```python
from build123d import *

# Parameters (mm, degrees)
SKETCH1_W           = 25.5
SKETCH1_H           = 4
BOSS_EXTRUDE1_DEPTH = 2
FILLET1_R           = 10
SKETCH2_R           = 1.5
CUT_EXTRUDE1_DEPTH  = 53.603569832
SKETCH3_W           = 29.5
SKETCH3_H           = 2
BOSS_EXTRUDE2_DEPTH = 5.1
SKETCH4_W           = 29.5
SKETCH4_H           = 3
BOSS_EXTRUDE3_DEPTH = 13.8
SKETCH5_W           = 29.5
SKETCH5_H           = 2
BOSS_EXTRUDE5_DEPTH = 34.8
SKETCH7_W           = 29.5
SKETCH7_H           = 2
BOSS_EXTRUDE6_DEPTH = 13.8
SKETCH8_W           = 2
SKETCH8_H           = 4
SKETCH8_H_2         = 6.1
BOSS_EXTRUDE7_DEPTH = 12
SKETCH9_2_R         = 1.25
CUT_EXTRUDE3_DEPTH  = 12
SKETCH9_R           = 1.25
CUT_EXTRUDE2_DEPTH  = 12


with BuildPart() as part:
    # Sketch1 → Boss-Extrude1 (new body)
    with BuildSketch(Plane(origin=(0, 0, 0), x_dir=(1, 0, 0), z_dir=(0, 1, 0))):
        Polygon((-37.234375, 16.8984375), (-41.234375, 16.8984375), (-41.234375, -32.6015625), (-37.234375, -32.6015625), (-37.234375, 12.8984375), align=None)
        with Locations((-24.484375, 14.8984375)):
            Rectangle(SKETCH1_W, SKETCH1_H)
    extrude(amount=BOSS_EXTRUDE1_DEPTH)

    # Fillet1
    fillet1_edges = [part.edges().sort_by_distance(p)[0] for p in [
        (-37.234375, 1, -12.8984375),
    ]]
    fillet(fillet1_edges, radius=FILLET1_R)

    # Sketch2 → Cut-Extrude1 (cut, through all)
    with BuildSketch(Plane(origin=(0, 2, 0), x_dir=(1, 0, 0), z_dir=(0, 1, 0))):
        with Locations(Location((-38.984375, -30.3515625, 0), (0, 0, 270))):
            Circle(SKETCH2_R)
        with Locations(Location((-38.984375, 14.6484375, 0), (0, 0, 270))):
            Circle(SKETCH2_R)
        with Locations(Location((-13.984375, 14.6484375, 0), (0, 0, 270))):
            Circle(SKETCH2_R)
    extrude(amount=-CUT_EXTRUDE1_DEPTH, mode=Mode.SUBTRACT)

    # Sketch3 → Boss-Extrude2 (add)
    with BuildSketch(Plane(origin=(0, 0, -16.8984375), x_dir=(-1, 0, 0), z_dir=(0, 0, -1))):
        with Locations((26.484375, 1)):
            Rectangle(SKETCH3_W, SKETCH3_H)
    extrude(amount=BOSS_EXTRUDE2_DEPTH)

    # Sketch4 → Boss-Extrude3 (add)
    with BuildSketch(Plane.XZ):
        with Locations((-26.484375, -20.4984375)):
            Rectangle(SKETCH4_W, SKETCH4_H)
    extrude(amount=BOSS_EXTRUDE3_DEPTH)

    # Sketch5 → Boss-Extrude5 (add)
    with BuildSketch(Plane(origin=(0, 0, -21.9984375), x_dir=(-1, 0, 0), z_dir=(0, 0, -1))):
        with Locations((26.484375, -12.8)):
            Rectangle(SKETCH5_W, SKETCH5_H)
    extrude(amount=BOSS_EXTRUDE5_DEPTH)

    # Sketch7 → Boss-Extrude6 (add)
    with BuildSketch(Plane(origin=(0, -11.8, 0), x_dir=(1, 0, 0), z_dir=(0, 1, 0))):
        with Locations((-26.484375, 55.7984375)):
            Rectangle(SKETCH7_W, SKETCH7_H)
    extrude(amount=BOSS_EXTRUDE6_DEPTH)

    # Sketch8 → Boss-Extrude7 (add)
    with BuildSketch(Plane(origin=(0, -11.8, 0), x_dir=(1, 0, 0), z_dir=(0, 1, 0))):
        with Locations((-12.734375, 23.9984375)):
            Rectangle(SKETCH8_W, SKETCH8_H)
        with Locations((-12.734375, 51.7484375)):
            Rectangle(SKETCH8_W, SKETCH8_H_2)
    extrude(amount=BOSS_EXTRUDE7_DEPTH)

    # Sketch9_2 → Cut-Extrude3 (cut)
    with BuildSketch(Plane(origin=(-11.734375, 0, 0), x_dir=(0, 0, -1), z_dir=(1, 0, 0))):
        with Locations((23.4984375, -5.55)):
            Circle(SKETCH9_2_R)
        with Locations((51.1984375, -5.55)):
            Circle(SKETCH9_2_R)
    extrude(amount=-CUT_EXTRUDE3_DEPTH, mode=Mode.SUBTRACT)

    # Sketch9 → Cut-Extrude2 (cut)
    with BuildSketch(Plane(origin=(-11.734375, 0, 0), x_dir=(0, 0, -1), z_dir=(1, 0, 0))):
        with Locations((23.4984375, -5.55)):
            Circle(SKETCH9_R)
        with Locations((51.1984375, -5.55)):
            Circle(SKETCH9_R)
    extrude(amount=-CUT_EXTRUDE2_DEPTH, mode=Mode.SUBTRACT)


solid = part.part
```
The listing builds one solid part. Answer for the finished solid, in the listing's coordinates (mm). A direction names the side the tool comes from. Round coordinates to 2 decimals unless told otherwise and drop trailing zeros. Loops run counter-clockwise (first coordinate to the right, second up) from the corner with the lowest first, then second, coordinate; pieces in that order, holes last. Notation, with made-up numbers: (-19, -3) -> (29, -3) arc R14 cw to (29, 15) -> close; hole circle Ø4 at (86.5, -17). An arc over 180 degrees is marked (long way). Use one line per item in the form item = value.
1. The part is cut by section D-D on x = -28.75. Determine the outline of the cut face in (y, z), and give its area (3 significant figures).
Answer key:
outline = (-13.8, -56.8) -> (2, -56.8) -> (2, -54.8) -> (-11.8, -54.8) -> (-11.8, -22) -> (2, -22) -> (2, -12.78) -> (0, -12.78) -> (0, -19) -> (-13.8, -19) -> close
area = 157 mm²
2. The part is cut by section C-C on z = -32. Determine the outline of the cut face in (x, y).
Answer key:
outline = (-41.23, -13.8) -> (-11.73, -13.8) -> (-11.73, -11.8) -> (-41.23, -11.8) -> close
3. Flat-ended cylindrical pins translate along their axes: pin 1 Ø3.5 at (x, z) = (-13.98, -14.65) entering from -Y; pin 2 Ø1.6 at (x, y) = (-19.5, 1.5) entering from +Z; pin 3 Ø0.6 at (x, y) = (-12.5, -4.5) entering from +Z. Find the tip coordinate at first contact, or state that the pin passes through.
Answer key:
pin_1 = 0
pin_2 = -12.9
pin_3 = -19
4. The part is cut by section A-A on y = -8.75. Determine the outline of the cut face in (x, z), and give its area (3 significant figures).
Answer key:
outline = (-41.23, -56.8) -> (-11.73, -56.8) -> (-11.73, -48.7) -> (-13.73, -48.7) -> (-13.73, -54.8) -> (-41.23, -54.8) -> close; (-41.23, -22) -> (-13.73, -22) -> (-13.73, -26) -> (-11.73, -26) -> (-11.73, -19) -> (-41.23, -19) -> close
area = 168 mm²
5. Find the intervals of material crossed by probe 1 along Z at (x, y) = (-33, -4); probe 2 along Y at (x, z) = (-34, -15), in increasing order. Write a range as [from, to].
Answer key:
probe_1 = [-56.8, -54.8], [-22, -19]
probe_2 = [0, 2]
6. For a pull along Z with two mould halves and no side action, classify faces 1 (the flat face through (-13.734, -6, -25)), 2 (the flat face through (-41.234, -4.2, -21.8)), 3 (the flat face through (-27, -6, -56.798)), 4 (the cylindrical face through (-34.383, 1.014, -9.891)) as released by +Z, released by -Z, zero draft, split by the parting line, or undercut.
Answer key:
face_1 = undercut
face_2 = zero draft
face_3 = released by -Z
face_4 = released by +Z
7. The part is cut by section B-B on x = -21.75. Determine the outline of the cut face in (y, z).
Answer key:
outline = (-13.8, -56.8) -> (2, -56.8) -> (2, -54.8) -> (-11.8, -54.8) -> (-11.8, -22) -> (2, -22) -> (2, -12.9) -> (0, -12.9) -> (0, -19) -> (-13.8, -19) -> close
8. A tool of negligible diameter and unlimited length cuts with its end or side. For faces 5 (the flat face through (-13, 0.2, -52)), 6 (the flat face through (-13.734, -7, -52)), 7 (the flat face through (-37.234, 1, 15)), 8 (the flat face through (-38, 0, -3)), from which of +Z, -Z, +X, -X, +Y, -Y can it reach the whole face along a straight path? Write none if from no direction.
Answer key:
face_5 = +X, -X, +Y
face_6 = -X, +Y
face_7 = +Z, +X, +Y, -Y
face_8 = +Z, +X, -X, -Y
